```python
from build123d import *

# Parameters (mm, degrees)
F0_R           = 6.5
F0_R_2         = 6.1
F1_DEPTH       = 3
F3_D           = 3.5
F3_CBORE_D     = 6.5
F3_CBORE_DEPTH = 2


with BuildPart() as f1:
    # F0 (on Front) → F1 (new body)
    with BuildSketch(Plane.XZ):
        with BuildLine():
            Line((-91, -40), (91, -40))
            ThreePointArc((91, -40), (93.828427, -38.828427), (95, -36))
            Line((95, -36), (95, 36))
            ThreePointArc((95, 36), (93.828427, 38.828427), (91, 40))
            Line((91, 40), (-91, 40))
            ThreePointArc((-91, 40), (-93.828427, 38.828427), (-95, 36))
            Line((-95, 36), (-95, -36))
            ThreePointArc((-95, -36), (-93.828427, -38.828427), (-91, -40))
        make_face()
        with Locations((-45, 0)):
            Circle(F0_R, mode=Mode.SUBTRACT)
        with Locations((-5, 0)):
            Circle(F0_R, mode=Mode.SUBTRACT)
        with Locations((65, 0)):
            Circle(F0_R_2, mode=Mode.SUBTRACT)
    extrude(amount=-F1_DEPTH)

    # F3 (through all)
    with Locations(Plane(origin=(0, 3, 0), x_dir=(-1, 0, 0), z_dir=(0, 1, 0))):
        with Locations((-90, 35), (90, 35), (90, -35), (-90, -35)):
            CounterBoreHole(F3_D / 2, F3_CBORE_D / 2, F3_CBORE_DEPTH)


solid = f1.part
```
For this review, take the finished solid that the model builds, in its own axes (mm). A direction names the side the tool comes from. Coordinates: 2 decimals unless noted, no trailing zeros. Order: outer loops, then holes, each group sorted by start corner. A loop starts at its lowest first (then second) coordinate and runs counter-clockwise, first axis right, second up. Notation, with made-up numbers: (6, 0.5) -> (54, 0.5) arc R21 cw to (54, 12.5) -> close; hole circle Ø6 at (6, 69). An arc over 180 degrees is marked (long way). Use CSV: the item, a comma, the result in double quotes. Start each with the question number.
Item 1: We need section A-A, the plane x = -45. Give the boundary of the cut face in (y, z).
Item 2: For faces 1 (the face through (88.6, 1, 33.6)), 2 (the face through (-88.331, 0.493, -34.474)), list the 3-axis set-ups (+Z, -Z, +X, -X, +Y, -Y) from which the entire face can be reached by the end or side of a thin tool; tool diameter is ignored.
Item 3: Insertion check: pin 1 (6 mm diameter, centred on x = -90, z = 35, fed in from +Y); pin 2 (21 mm diameter, centred on x = -5, z = 0, fed in from -Y). Each pin has a flat end and moves straight along its axis. Give the tip position at first contact, or say it passes through.
Item 4: We need section C-C, the plane y = 2. Give the boundary of the cut face in (x, z).
Item 5: Wall thickness on probe 1 along Z at (x, y) = (-90, 0.65); probe 2 along Z at (x, y) = (90, 2.55); probe 3 along X at (y, z) = (2.45, 5): over which ranges is each line inside the solid? List them lowest first.
Item 6: We need section B-B, the plane z = 0. Give the boundary of the cut face in (x, y).
Item 7: We need section D-D, the plane x = 65. Give the boundary of the cut face in (y, z), then the cut area to 3 significant figures.
Item 8: Draft analysis for pull direction Z (two halves, no side actions). For faces 3 (the face through (89.62, 0.49, 33.29)), 4 (the face through (-93.859, 1.479, -38.797)), 5 (the face through (-1, 3, 9)), state which applies: pulls with the +Z half, pulls with the -Z half, needs draft (parallel to the pull), parting line crosses it, or undercut.
Derived:
1,outline,"(0, -40) -> (3, -40) -> (3, -6.5) -> (0, -6.5) -> close; (0, 6.5) -> (3, 6.5) -> (3, 40) -> (0, 40) -> close"
2,face 1,"+Y"
2,face 2,"+Y, -Y"
3,pin 1,"stops at y = 1"
3,pin 2,"stops at y = 0"
4,outline,"(-95, -36) arc R4 ccw to (-91, -40) -> (91, -40) arc R4 ccw to (95, -36) -> (95, 36) arc R4 ccw to (91, 40) -> (-91, 40) arc R4 ccw to (-95, 36) -> close; hole circle Ø6.5 at (-90, -35); hole circle Ø6.5 at (-90, 35); hole circle Ø13 at (-45, 0); hole circle Ø13 at (-5, 0); hole circle Ø12.2 at (65, 0); hole circle Ø6.5 at (90, -35); hole circle Ø6.5 at (90, 35)"
5,probe 1,"z = -40 to -36.75, -33.25 to 33.25, 36.75 to 40"
5,probe 2,"z = -40 to -38.25, -31.75 to 31.75, 38.25 to 40"
5,probe 3,"x = -95 to -49.15, -40.85 to -9.15, -0.85 to 61.51, 68.49 to 95"
6,outline,"(-95, 0) -> (-51.5, 0) -> (-51.5, 3) -> (-95, 3) -> close; (-38.5, 0) -> (-11.5, 0) -> (-11.5, 3) -> (-38.5, 3) -> close; (1.5, 0) -> (58.9, 0) -> (58.9, 3) -> (1.5, 3) -> close; (71.1, 0) -> (95, 0) -> (95, 3) -> (71.1, 3) -> close"
7,outline,"(0, -40) -> (3, -40) -> (3, -6.1) -> (0, -6.1) -> close; (0, 6.1) -> (3, 6.1) -> (3, 40) -> (0, 40) -> close"
7,area,"203 mm^2"
8,face 3,"undercut"
8,face 4,"pulls with the -Z half"
8,face 5,"needs draft"
